Can you work these out from the drawing? Everything is in mm from the part's minimum corner. Give positions to 0.01 mm unless a question says otherwise; leave off trailing zeros. Loops run counter-clockwise (first coordinate to the right, second up) from the corner with the lowest first, then second, coordinate; pieces in that order, holes last.
Q1. If we section it at C-C (x = 38.1): Please give me the cut outline in (y, z), plus the area to 3 significant figures.
Q2. I need wall thicknesses on line 1 (Z direction, x = 38.1, y = 13); line 2 (X direction, y = 14.25, z = 9); line 3 (X direction, y = 10.5, z = 3.75). Which ranges of each line are inside material? Lowest first, please.
Q3. Will this pin go through, and if not, where does the flat tip stop? P1, Ø10, axis at y = 3.5, z = 3, coming from the -X side.
Q4. We'd pull the mould along Z, two halves only. Please class the marked faces 1, 2 and 3: +Z half, -Z half, draft (parallel to the pull), parting line (faces both ways), or undercut.
Q5. If we section it at A-A (y = 8): Give the number of separate pieces and of enclosed holes in the cut face, plus the area to 3 significant figures.
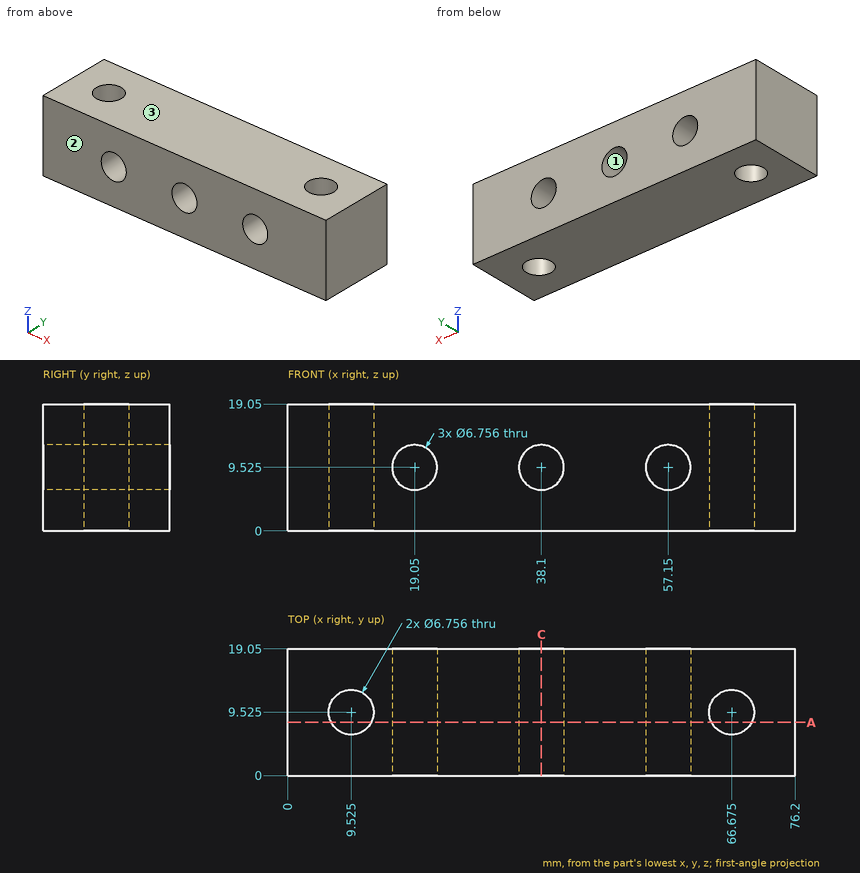
Check sheet entries:
1. outline: (0, 0) - (19.05, 0) - (19.05, 6.15) - (0, 6.15) - close; (0, 12.9) - (19.05, 12.9) - (19.05, 19.05) - (0, 19.05) - close
1. area: 234 mm2
2. line 1: z = 0 to 6.15, 12.9 to 19.05
2. line 2: x = 0 to 15.71, 22.39 to 34.76, 41.44 to 53.81, 60.49 to 76.2
2. line 3: x = 0 to 6.29, 12.76 to 63.44, 69.91 to 76.2
3. P1: stops at x = 0
4. face 1: undercut
4. face 2: draft
4. face 3: +Z half
5. separate pieces: 3
5. enclosed holes: 3
5. area: 1,110 mm2
